```python
from build123d import *

# Parameters (mm, degrees)
BOSS_EXTRUDE1_DEPTH = 3
SKETCH2_R           = 2.5
CUT_EXTRUDE1_DEPTH  = 5
FILLET1_R           = 5


with BuildPart() as part:
    # Sketch1 → Boss-Extrude1 (new body)
    with BuildSketch(Plane(origin=(0, 0, 0), x_dir=(1, 0, 0), z_dir=(0, 1, 0))):
        Polygon((0, 0), (73.5, 0), (73.5, -35), (93.3, -35), (93.3, 0), (166.8, 0), (166.8, 274.8), (0, 274.8), align=None)
    extrude(amount=BOSS_EXTRUDE1_DEPTH)

    # Sketch2 → Cut-Extrude1 (cut)
    with BuildSketch(Plane(origin=(0, 3, 0), x_dir=(1, 0, 0), z_dir=(0, 1, 0))):
        with Locations(Location((83.4, -30, 0), (0, 0, 270))):
            Circle(SKETCH2_R)
    extrude(amount=-CUT_EXTRUDE1_DEPTH, mode=Mode.SUBTRACT)

    # Fillet1
    fillet1_edges = [part.edges().sort_by_distance(p)[0] for p in [
        (0, 1.5, -274.8),
        (166.8, 1.5, -274.8),
        (166.8, 1.5, 0),
        (93.3, 1.5, 35),
        (73.5, 1.5, 35),
        (0, 1.5, 0),
    ]]
    fillet(fillet1_edges, radius=FILLET1_R)


solid = part.part
```
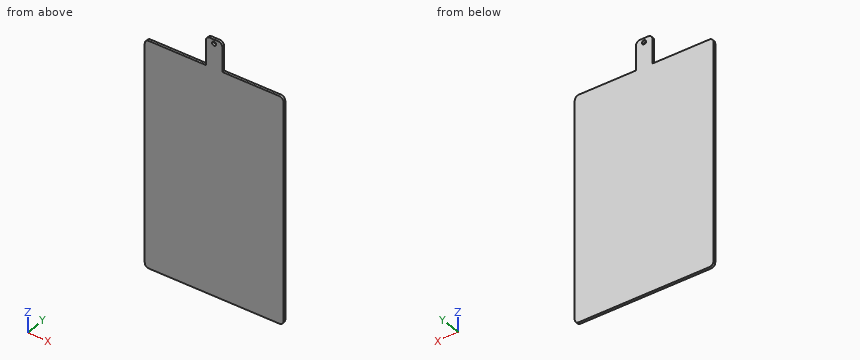
Part model, mm, in its own coordinate system. Coordinates: 2 decimals unless noted, no trailing zeros. Order: outer loops, then holes, each group sorted by start corner. A loop starts at its lowest first (then second) coordinate and runs counter-clockwise, first axis right, second up. Notation, with made-up numbers: (58.5, -18.5) -> (95.5, -18.5) arc R28 cw to (95.5, 15.5) -> close; hole circle Ø4 at (21.25, 52.25). An arc over 180 degrees is marked (long way). Put each result on its own line as item: value. Start each with the question number.
(1) Band-saw the part on B-B (x = 37). Give the cut face in (y, z), then the cut area to 3 significant figures.
(2) Probe line 1 along X through (y, z) = (1.95, 30); line 2 along Z through (x, y) = (23, 2.6); line 3 along X through (y, z) = (2.65, -4.5). List the from-to ranges inside material, lowest first. Write a range as [from, to].
(3) Band-saw the part on A-A (y = 1.6). Give the cut face in (x, z).
(4) Pin check, flat tips, straight feed: pin 1 Ø1.5 at (x, z) = (74.5, -120) entering from -Y; pin 2 Ø1.5 at (y, z) = (1.5, 16) entering from -X. Stop position of each tip, or through.
Determined:
1. outline: (0, -274.8) -> (3, -274.8) -> (3, 0) -> (0, 0) -> close
1. area: 824 mm²
2. line 1: x = [73.5, 80.9], [85.9, 93.3]
2. line 2: z = [-274.8, 0]
2. line 3: x = [0.03, 166.77]
3. outline: (0, -269.8) arc R5 ccw to (5, -274.8) -> (161.8, -274.8) arc R5 ccw to (166.8, -269.8) -> (166.8, -5) arc R5 ccw to (161.8, 0) -> (93.3, 0) -> (93.3, 30) arc R5 ccw to (88.3, 35) -> (78.5, 35) arc R5 ccw to (73.5, 30) -> (73.5, 0) -> (5, 0) arc R5 ccw to (0, -5) -> close; hole circle Ø5 at (83.4, 30)
4. pin 1: stops at y = 0
4. pin 2: stops at x = 73.5
